Study the drawing (mm; zero at the part's minimum x, y, z) and answer. Coordinates: 2 decimals unless noted, no trailing zeros. Write each loop counter-clockwise with the first axis right and the second up, starting at its lowest first coordinate (ties: lowest second). Pieces come first, ordered by that corner, then holes. Notation, with made-up numbers: (82.5, 12.25) - (133.5, 12.25) arc R17 ccw to (133.5, 32.25) - close; hole circle Ø2 at (88.5, 2.5). An arc over 180 degrees is marked (long way). One line per item, written item: value.
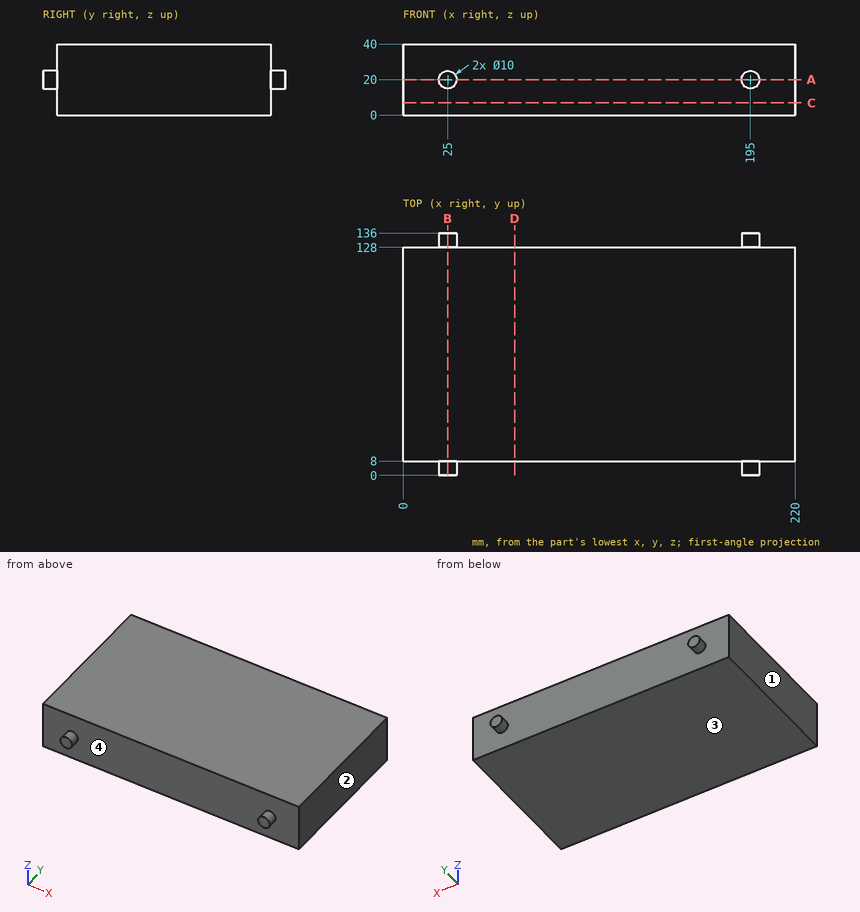
Item 1: Given pin 1 (20 mm diameter, centred on x = 82, z = 13.5, fed in from +Y); pin 2 (2 mm diameter, centred on x = 101.5, z = 23, fed in from -Y), each flat-ended and moving along its own axis, determine where each tip first touches the part or whether it passes through.
Evaluation:
pin 1: stops at y = 128
pin 2: stops at y = 8
Item 2: Section C-C, the plane z = 7 is taken. Determine the outline of the cut face in (x, y).
Evaluation:
outline: (0, 8) - (220, 8) - (220, 128) - (0, 128) - close
Item 3: Determine the mould class of the marked faces 1, 2, 3 and 4 for opening direction X: +X half, -X half, draft (parallel to the pull), parting line (faces both ways), or undercut.
Evaluation:
face 1: -X half
face 2: +X half
face 3: draft
face 4: undercut
Item 4: Section A-A, the plane z = 20 is taken. Determine the outline of the cut face in (x, y).
Evaluation:
outline: (0, 8) - (20, 8) - (20, 0) - (30, 0) - (30, 8) - (190, 8) - (190, 0) - (200, 0) - (200, 8) - (220, 8) - (220, 128) - (200, 128) - (200, 136) - (190, 136) - (190, 128) - (30, 128) - (30, 136) - (20, 136) - (20, 128) - (0, 128) - close
Item 5: Consider probe 1 along Y at (x, z) = (121, 18); probe 2 along X at (y, z) = (6, 15.5); probe 3 along X at (y, z) = (7.5, 19). Determine where each line is inside the solid, lowest interval first.
Evaluation:
probe 1: y = 8 to 128
probe 2: x = 22.82 to 27.18, 192.82 to 197.18
probe 3: x = 20.1 to 29.9, 190.1 to 199.9
Item 6: Section D-D, the plane x = 62.5 is taken. Determine the outline of the cut face in (y, z), then the cut area to 3 significant figures.
Evaluation:
outline: (8, 0) - (128, 0) - (128, 40) - (8, 40) - close
area: 4,800 mm2
Item 7: Section B-B, the plane x = 25 is taken. Determine the outline of the cut face in (y, z).
Evaluation:
outline: (0, 15) - (8, 15) - (8, 0) - (128, 0) - (128, 15) - (136, 15) - (136, 25) - (128, 25) - (128, 40) - (8, 40) - (8, 25) - (0, 25) - close
